Input: part model. Units: mm. Frame: model coordinates. Give positions to 0.01 mm unless a question says otherwise; leave off trailing zeros. Write each loop counter-clockwise with the first axis right and the second up, starting at its lowest first coordinate (ties: lowest second). Pieces come first, ordered by that corner, then holes. Notation, with made-up numbers: (62, 66) - (88, 66) arc R26 ccw to (88, 88) - close; hole circle Ø7 at (-22, 47). An arc over 180 degrees is marked (long way). Use a Markdown table: item, result. Add a question column.
1. Section query B-B, the plane x = -2. Return loops of the section in (y, z).
2. Pin query (flat end, axial travel): pin 1 (10 mm diameter, centred on x = -69, y = 31.5, fed in from -Z). Return the tip coordinate at first contact, or that it passes through.
3. Material intervals for probe 1 along Y at (x, z) = (50, 1.4); probe 2 along Y at (x, z) = (-20, 3.65); probe 3 along X at (y, z) = (32, 1), sorted ascending.
4. Section query C-C, the plane z = 2.95. Return loops of the section in (x, y), plus the area to 3 significant figures.
5. Section query A-A, the plane y = 6.5. Return loops of the section in (x, z).
```python
from build123d import *

# Parameters (mm, degrees)
F0_W     = 166
F0_H     = 100.4
F1_DEPTH = 4
F0_W_2   = 155
F0_H_2   = 87.6
F2_DEPTH = 2
F3_SIZE  = 1


with BuildPart() as f1:
    # F0 (on Top) → F1 (new body)
    with BuildSketch(Plane.XY):
        Polygon((97.986992, 48.91296), (-92.013008, 48.91296), (-92.013008, -67.28704), (-79.013008, -67.28704), (-79.013008, -66.73704), (-72.013008, -66.73704), (-72.013008, -67.28704), (77.986992, -67.28704), (77.986992, -66.73704), (84.986992, -66.73704), (84.986992, -67.28704), (97.986992, -67.28704), align=None)
        with Locations((4.986992, -7.68704)):
            Rectangle(F0_W, F0_H, mode=Mode.SUBTRACT)
    extrude(amount=F1_DEPTH)

    # F0 (on Top) → F2 (join)
    with BuildSketch(Plane.XY):
        with Locations((4.986992, -7.68704)):
            Rectangle(F0_W, F0_H)
        with Locations((2.986992, -9.18704)):
            Rectangle(F0_W_2, F0_H_2, mode=Mode.SUBTRACT)
    extrude(amount=F2_DEPTH)

    # F3
    f3_edges = [f1.edges().sort_by_distance(p)[0] for p in [
        (2.986992, -52.98704, 0),
        (-74.513008, -9.18704, 0),
        (2.986992, 34.61296, 0),
        (80.486992, -9.18704, 0),
    ]]
    chamfer(f3_edges, length=F3_SIZE)


solid = f1.part
```
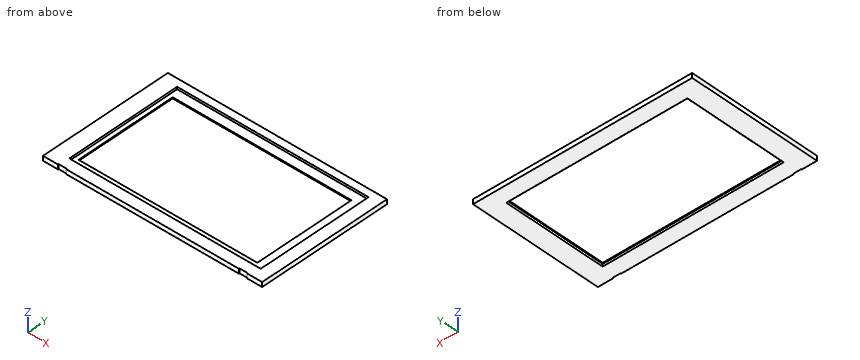
Result sheet:
| question | item | result |
|---|---|---|
| 1 | outline | (-67.29, 0) - (-53.99, 0) - (-52.99, 1) - (-52.99, 2) - (-57.89, 2) - (-57.89, 4) - (-67.29, 4) - close; (34.61, 1) - (35.61, 0) - (48.91, 0) - (48.91, 4) - (42.51, 4) - (42.51, 2) - (34.61, 2) - close |
| 2 | pin 1 | stops at z = 0 |
| 3 | probe 1 | y = -67.29 to -52.99, 34.61 to 48.91 |
| 3 | probe 2 | y = -67.29 to -57.89, 42.51 to 48.91 |
| 3 | probe 3 | x = -92.01 to -74.51, 80.49 to 97.99 |
| 4 | outline | (-92.01, -67.29) - (-79.01, -67.29) - (-79.01, -66.74) - (-72.01, -66.74) - (-72.01, -67.29) - (77.99, -67.29) - (77.99, -66.74) - (84.99, -66.74) - (84.99, -67.29) - (97.99, -67.29) - (97.99, 48.91) - (-92.01, 48.91) - close; hole (-78.01, -57.89) - (87.99, -57.89) - (87.99, 42.51) - (-78.01, 42.51) - close |
| 4 | area | 5,400 mm² |
| 5 | outline | (-92.01, 0) - (-75.51, 0) - (-74.51, 1) - (-74.51, 2) - (-78.01, 2) - (-78.01, 4) - (-92.01, 4) - close; (80.49, 1) - (81.49, 0) - (97.99, 0) - (97.99, 4) - (87.99, 4) - (87.99, 2) - (80.49, 2) - close |
